from build123d import *

# Parameters (mm, degrees)
SKETCH1_W               = 25.4
SKETCH1_H               = 25.4
SKETCH1_W_2             = 19.05
SKETCH1_H_2             = 19.05
BOSS_EXTRUDE1_DEPTH     = 279.4
CUT_EXTRUDE1_DEPTH      = 282.699627263
CUT_EXTRUDE1_DEPTH_BACK = 282.699627263
SKETCH2_R               = 3.175
F_10_CLEARANCE_HOLE1_D  = 5.1054


with BuildPart() as part:
    # Sketch1 → Boss-Extrude1 (new body)
    with BuildSketch(Plane.XY):
        with Locations((-12.7, 12.7)):
            Rectangle(SKETCH1_W, SKETCH1_H)
        with Locations((-12.7, 12.7)):
            Rectangle(SKETCH1_W_2, SKETCH1_H_2, mode=Mode.SUBTRACT)
    extrude(amount=BOSS_EXTRUDE1_DEPTH)

    # Sketch2 → Cut-Extrude1 (cut, two sides: drawn at the far end of the back side and taken through both)
    with BuildSketch(Plane(origin=(0, 0, 0), x_dir=(-1, 0, 0), z_dir=(0, -1, 0)).offset(-CUT_EXTRUDE1_DEPTH_BACK)):
        with Locations(Location((12.7, -266.7, 0), (0, 0, 90))):
            Circle(SKETCH2_R)
    extrude(amount=CUT_EXTRUDE1_DEPTH + CUT_EXTRUDE1_DEPTH_BACK, mode=Mode.SUBTRACT)

    # #10 Clearance Hole1 (through all)
    with Locations(Plane(origin=(0, 25.4, 0), x_dir=(1, 0, 0), z_dir=(0, 1, 0))):
        with Locations((-12.7, -38.1), (-12.7, -25.4), (-12.7, -12.7)):
            Hole(F_10_CLEARANCE_HOLE1_D / 2)


solid = part.part
For this review, take the finished solid that the model builds, in its own axes (mm). A direction names the side the tool comes from. Give positions to 0.01 mm unless a question says otherwise; leave off trailing zeros. Order: outer loops, then holes, each group sorted by start corner. A loop starts at its lowest first (then second) coordinate and runs counter-clockwise, first axis right, second up. Notation, with made-up numbers: M 42,62 L 63,62 A9 cw 63,78 Z; hole C 45.5,80 d3. An arc over 180 degrees is marked long. Answer in a Markdown table with one row per item. Add a question column.
(1) Wall thickness on probe 1 along Z at (x, y) = (-12.7, 1.9) (3 decimals); probe 2 along X at (y, z) = (24, 266.7) (3 decimals); probe 3 along Y at (x, z) = (-5.25, 225) (3 decimals): over which ranges is each line inside the solid? List them lowest first. Write a range as [from, to].
(2) Consider section A-A on z = 266.7. State the section outline as (x, y) points (3 decimals).
(3) For faces 1 (the face through (-3.175, 13, 138)), 2 (the face through (-14.072, 23.79, 35.948)), list the 3-axis set-ups (+Z, -Z, +X, -X, +Y, -Y) from which the entire face can be reached by the end or side of a thin tool; tool diameter is ignored.
(4) Mouldability with a two-part tool opening along X and no side actions: class faces 3 (the face through (-2, 13, 279.4)), 4 (the face through (-15.058, 23.79, 26.378)), 5 (the face through (0, 13, 138)) as +X half, -X half, draft (parallel to the pull), parting line (faces both ways), or undercut.
(5) Consider section B-B on y = 6.5. State the section outline as (x, z) points (3 decimals).
(6) Consider section C-C on z = 12.7. State the section outline as (x, y) points (3 decimals).
(7) For pin 1 (9.5 mm diameter, centred on y = 11.5, z = 126, fed in from +X), flat-tipped, find the tip position at first contact; note if it passes through.
(8) Consider section D-D on z = 172. State the section outline as (x, y) points (3 decimals), and give its area (3 significant figures).
Evaluation:
| question | item | result |
|---|---|---|
| 1 | probe 1 | z = [0, 10.147], [15.253, 22.847], [27.953, 35.547], [40.653, 263.525], [269.875, 279.4] |
| 1 | probe 2 | x = [-25.4, -15.875], [-9.525, 0] |
| 1 | probe 3 | y = [0, 3.175], [22.225, 25.4] |
| 2 | outline | M -25.4,0 L -15.875,0 L -15.875,3.175 L -22.225,3.175 L -22.225,22.225 L -15.875,22.225 L -15.875,25.4 L -25.4,25.4 Z; M -9.525,0 L 0,0 L 0,25.4 L -9.525,25.4 L -9.525,22.225 L -3.175,22.225 L -3.175,3.175 L -9.525,3.175 Z |
| 3 | face 1 | +Z, -Z |
| 3 | face 2 | +Y, -Y |
| 4 | face 3 | draft |
| 4 | face 4 | undercut |
| 4 | face 5 | +X half |
| 5 | outline | M -25.4,0 L -22.225,0 L -22.225,279.4 L -25.4,279.4 Z; M -3.175,0 L 0,0 L 0,279.4 L -3.175,279.4 Z |
| 6 | outline | M -25.4,0 L -15.253,0 L -15.253,3.175 L -22.225,3.175 L -22.225,22.225 L -15.253,22.225 L -15.253,25.4 L -25.4,25.4 Z; M -10.147,0 L 0,0 L 0,25.4 L -10.147,25.4 L -10.147,22.225 L -3.175,22.225 L -3.175,3.175 L -10.147,3.175 Z |
| 7 | pin 1 | stops at x = 0 |
| 8 | outline | M -25.4,0 L 0,0 L 0,25.4 L -25.4,25.4 Z; hole M -22.225,3.175 L -3.175,3.175 L -3.175,22.225 L -22.225,22.225 Z |
| 8 | area | 282 mm^2 |
